Autodesk Inventor part; units mm, degrees
ref_plane "YZ Plane" through (0, 0, 0) normal (1, 0, 0) x (0, 1, 0)
ref_plane "XZ Plane" through (0, 0, 0) normal (0, 1, 0) x (-1, 0, 0)
ref_plane "XY Plane" through (0, 0, 0) normal (0, 0, 1) x (1, 0, 0)
sketch "Sketch1" plane through (0, 0, 0) normal (0, 0, 1) x (1, 0, 0)
  line L0 (-190.2533, 169.37) -> (-164.8533, 169.37)
  line L1 (165.3467, -186.23) -> (165.3467, -211.63)
  line L2 (165.3467, -211.63) -> (-190.2533, -211.63)
  line L3 (-190.2533, -211.63) -> (-190.2533, 169.37)
  line L4 (165.3467, -186.23) -> (-164.8533, -186.23)
  line L5 (-164.8533, -186.23) -> (-164.8533, -110.03)
  line L6 (-164.8533, -110.03) -> (139.9467, -110.03)
  line L7 (139.9467, -84.63) -> (-164.8533, -84.63)
  line L8 (-164.8533, -84.63) -> (-164.8533, -8.43)
  line L9 (-164.8533, -8.43) -> (101.8467, -8.43)
  line L10 (101.8467, -8.43) -> (101.8467, 16.97)
  line L11 (101.8467, 16.97) -> (-164.8533, 16.97)
  line L12 (-164.8533, 16.97) -> (-164.8533, 93.17)
  line L13 (-164.8533, 93.17) -> (38.3467, 93.17)
  line L14 (38.3467, 93.17) -> (38.3467, 118.57)
  line L15 (38.3467, 118.57) -> (-164.8533, 118.57)
  line L16 (-164.8533, 118.57) -> (-164.8533, 169.37)
  line L17 (139.9467, -84.63) -> (139.9467, -110.03)
  point P0 (0, 0)
  dimension "d0" = 381
  dimension "d1" = 355.6
  dimension "d2" = 25.4
  dimension "d3" = 25.4
  dimension "d5" = 25.4
  dimension "d6" = 25.4
  dimension "d7" = 25.4
  dimension "d8" = 76.2
  dimension "d9" = 76.2
  dimension "d10" = 76.2
  dimension "d11" = 203.2
  dimension "d12" = 266.7
  dimension "d13" = 304.8
extrude "Extrusion1" add sketch "Sketch1" along normal blind 25.4
fillet "Fillet1" radius 12.7 5 edges at (165.3467, -186.23, 12.7) (139.9467, -84.63, 12.7) (139.9467, -110.03, 12.7) (101.8467, 16.97, 12.7) (101.8467, -8.43, 12.7)
fillet "Fillet1" radius 12.7 2 edges at (38.3467, 118.57, 12.7) (38.3467, 93.17, 12.7)
fillet "Fillet2" radius 6.35 6 edges at (34.6271, 114.8504, 25.4) (-69.6031, 93.17, 25.4) (-69.6031, 118.57, 25.4) (34.6271, 114.8504, 0) (-69.6031, 93.17, 0) (-69.6031, 118.57, 0)
fillet "Fillet3" radius 6.35 26 edges at (-164.8533, 143.97, 25.4) (-164.8533, 143.97, 0) (-164.8533, 55.07, 25.4) (-164.8533, 55.07, 0) (98.1271, 13.2504, 25.4) (-37.8531, -8.43, 25.4) (-37.8531, 16.97, 25.4) (98.1271, 13.2504, 0) (-37.8531, -8.43, 0) (-37.8531, 16.97, 0) (-164.8533, -46.53, 25.4) (-164.8533, -46.53, 0) (136.2271, -88.3496, 25.4) (-18.8031, -84.63, 25.4) (-18.8031, -110.03, 25.4) (136.2271, -88.3496, 0) (-18.8031, -110.03, 0) (-18.8031, -84.63, 0) (-164.8533, -148.13, 25.4) (-164.8533, -148.13, 0) (161.6271, -189.9496, 25.4) (165.3467, -205.2798, 25.4) (-6.1031, -186.23, 25.4) (161.6271, -189.9496, 0) (165.3467, -205.2798, 0) (-6.1031, -186.23, 0)
properties part number "snowboard rack" material "Wood (Birch)"
CAD build for the part. Positions are in the model's coordinates, mm. A direction names the side the tool comes from. Coordinates: 2 decimals unless noted, no trailing zeros. Order: outer loops, then holes, each group sorted by start corner. A loop starts at its lowest first (then second) coordinate and runs counter-clockwise, first axis right, second up.
Item 1: Band-saw the part on B-B on x = -55.5. Give the number of separate pieces and of enclosed holes in the cut face, plus the area to 3 significant figures.
Check sheet entries:
separate pieces: 4
enclosed holes: 0
area: 2,460 mm2
Item 2: Pin check, flat tips, straight feed: pin 1 Ø4 at (y, z) = (-40.5, 9.5) entering from +X; pin 2 Ø14 at (x, z) = (21.5, 10.5) entering from +Y; pin 3 Ø5 at (y, z) = (-6, 11.5) entering from +X. Stop position of each tip, or through.
Check sheet entries:
pin 1: stops at x = -164.85
pin 2: stops at y = 118.57
pin 3: stops at x = 99.19
Item 3: Drill centre lines: L1, parallel to Y at x = 10.5, z = 6.75; L2, parallel to Y at x = 79.5, z = 11.5; L3, parallel to Y at x = -38.5, z = 20. Where is each one in solid material? Low to high.
Check sheet entries:
L1: y = -211.63 to -186.23, -110.03 to -84.63, -8.43 to 16.97, 93.17 to 118.57
L2: y = -211.63 to -186.23, -110.03 to -84.63, -8.43 to 16.97
L3: y = -211.63 to -186.3, -109.96 to -84.7, -8.36 to 16.9, 93.24 to 118.5
Item 4: Two-plate mould, pull along Y, no slides. Class faces 4 (the face through (136.128, -106.409, 12.789)), 5 (the face through (-107, 8, 25.4)), 6 (the face through (-36, 16.97, 13)), 7 (the face through (34.725, 114.751, 12.789)): +Y half, -Y half, draft (parallel to the pull), parting line (faces both ways), or undercut.
Check sheet entries:
face 4: undercut
face 5: draft
face 6: undercut
face 7: +Y half
Item 5: 3-axis set-ups, long thin cutter, end or side, ignore diameter. For faces 1 (the face through (34.528, 96.791, 12.789)), 2 (the face through (-10, -211.63, 13)), 3 (the face through (-164.853, 144, 13)): which of +Z, -Z, +X, -X, +Y, -Y reach the whole face in a straight line?
Check sheet entries:
face 1: +Z, -Z, +X
face 2: +Z, -Z, +X, -X, -Y
face 3: +Z, -Z, +X, +Y
Item 6: Band-saw the part on D-D on y = 42. List the corners of the cut face in (x, z), plus the area to 3 significant figures.
Check sheet entries:
outline: (-190.25, 0) - (-171.2, 0) arc R6.35 ccw to (-164.85, 6.35) - (-164.85, 19.05) arc R6.35 ccw to (-171.2, 25.4) - (-190.25, 25.4) - close
area: 628 mm2
Item 7: Band-saw the part on A-A on x = 81. List the corners of the cut face in (y, z), plus the area to 3 significant figures.
Check sheet entries:
outline: (-211.63, 0) - (-192.58, 0) arc R6.35 ccw to (-186.23, 6.35) - (-186.23, 19.05) arc R6.35 ccw to (-192.58, 25.4) - (-211.63, 25.4) - close; (-110.03, 6.35) arc R6.35 ccw to (-103.68, 0) - (-90.98, 0) arc R6.35 ccw to (-84.63, 6.35) - (-84.63, 19.05) arc R6.35 ccw to (-90.98, 25.4) - (-103.68, 25.4) arc R6.35 ccw to (-110.03, 19.05) - close; (-8.43, 6.35) arc R6.35 ccw to (-2.08, 0) - (10.62, 0) arc R6.35 ccw to (16.97, 6.35) - (16.97, 19.05) arc R6.35 ccw to (10.62, 25.4) - (-2.08, 25.4) arc R6.35 ccw to (-8.43, 19.05) - close
area: 1,850 mm2
